CAD build for the part. Positions are in the model's coordinates, mm. Face numbers are marked on the shaded views. A direction names the side the tool comes from. Round coordinates to 2 decimals unless told otherwise and drop trailing zeros. Write each loop counter-clockwise with the first axis right and the second up, starting at its lowest first coordinate (ties: lowest second). Pieces come first, ordered by that corner, then holes. Notation, with made-up numbers: (83.5, 20) - (121.5, 20) arc R28 ccw to (121.5, 46) - close; hole circle Ø2 at (-11.5, 18). An arc over 180 degrees is marked (long way). Answer in a Markdown table with one row per item.
Autodesk Inventor part; units mm, degrees
ref_plane "YZ Plane" through (0, 0, 0) normal (1, 0, 0) x (0, 1, 0)
ref_plane "XZ Plane" through (0, 0, 0) normal (0, 1, 0) x (-1, 0, 0)
ref_plane "XY Plane" through (0, 0, 0) normal (0, 0, 1) x (1, 0, 0)
sketch "Szkic3" plane through (0, 0, 0) normal (0, 1, 0) x (-1, 0, 0)
  line L0 (3.9, 2.7912) -> (3.9, -2.7912)
  line L1 (6.5152, 5.4063) -> (3.9, 2.7912)
  line L2 (8.1306, 5.4063) -> (6.5152, 5.4063)
  line L3 (8.1306, 5.4063) -> (8.1306, 3.0781)
  line L4 (8.1306, -3.0781) -> (8.1306, -5.4064)
  line L5 (8.1306, -5.4064) -> (6.5152, -5.4064)
  line L6 (6.5152, -5.4064) -> (3.9, -2.7912)
  line L7 (8.1306, 3.0781) -> (8.5306, 3.0781)
  line L8 (8.1306, -3.0781) -> (8.5306, -3.0781)
  line L9 (8.5306, -3.0781) -> (12.0661, -6.6136)
  line L10 (8.5306, 3.0781) -> (12.0661, 6.6136)
  line L11 (12.0661, -6.6136) -> (12.0661, -12.6136)
  line L12 (12.0661, 6.6136) -> (12.0661, 12.6136)
  line L13 (12.0661, 12.6136) -> (16.0661, 12.6136)
  line L14 (12.0661, -12.6136) -> (16.0661, -12.6136)
  line L15 (16.0661, -12.6136) -> (16.0661, 12.6136)
  point P0 (8.1306, 4.2422)
  dimension "d85" = 5.5823
  dimension "d88" = 135
  dimension "d89" = 135
  dimension "d90" = 1.6154
  dimension "d91" = 2.6152
  dimension "d92" = 2.3282
  dimension "d99" = 0.4
  dimension "d100" = 5
  dimension "d101" = 135
  dimension "d102" = 5
  dimension "d103" = 135
  dimension "d114" = 180
  dimension "d115" = 6
  dimension "d116" = 6
  dimension "d117" = 4
  dimension "d118" = 4
extrude "Wyciągnięcie proste1" add sketch "Szkic3" along normal blind 24
sketch "Szkic13" plane through (-16.0661, 0, -12.6136) normal (-1, 0, 0) x (0, 0, 1)
  line L0 (12.6136, 15.06) -> (15.2636, 13.53)
  line L1 (15.2636, 13.53) -> (15.2636, 10.47)
  line L2 (15.2636, 10.47) -> (12.6136, 8.94)
  line L3 (12.6136, 8.94) -> (9.9636, 10.47)
  line L4 (9.9636, 10.47) -> (9.9636, 13.53)
  line L5 (9.9636, 13.53) -> (12.6136, 15.06)
  line L6 (0, 24) -> (25.2273, 24)
  line L7 (25.2273, 0) -> (25.2273, 24)
  point P0 (12.6136, 0)
  point P1 (12.6136, 12)
  point P2 (12.6136, 24)
  dimension "d119" = 12
  dimension "d120" = 12.6136
  dimension "d121" = 5.3
extrude "Wyciągnięcie proste5" cut sketch "Szkic13" against normal blind 6
sketch "Szkic14" plane through (-10.0661, 0, -12.6136) normal (-1, 0, 0) x (0, 0, 1)
  circle A0 centre (12.6136, 12) radius 1.7
  point P0 (12.6136, 0)
  dimension "d124" = 3.4
extrude "Wyciągnięcie proste6" cut sketch "Szkic14" against normal through all
sketch "Szkic15" plane through (0, 0, 0) normal (0, 0, 1) x (1, 0, 0)
  line L0 (-3.9, 13.7) -> (-3.9, 10.3)
  line L1 (-10.0661, 10.3) -> (-10.0661, 13.7)
  point P0 (0, 0)
  dimension "d127" = 6.1661
sketch "Szkic16" plane through (-16.0661, 0, -12.6136) normal (-1, 0, 0) x (0, 0, 1)
  point P0 (12.6136, 0)
sketch "Szkic17" plane through (-16.0661, 0, -12.6136) normal (-1, 0, 0) x (0, 0, 1)
  line L0 (25.2273, 0) -> (25.2273, 24)
  line L1 (0, 24) -> (25.2273, 24)
  line L2 (25.2273, 0) -> (18.7273, 0)
  line L3 (18.7273, 0) -> (18.7273, 24)
  line L4 (18.7273, 24) -> (25.2273, 24)
  line L5 (25.2273, 24) -> (25.2273, 0)
  line L6 (9.5355, 24) -> (6, 24)
  line L7 (6.5, 24) -> (0, 24)
  line L8 (0, 24) -> (0, 0)
  line L9 (0, 0) -> (6.5, 0)
  line L10 (6.5, 0) -> (6.5, 24)
  line L11 (0, 0) -> (0, 24)
  line L12 (0, 0) -> (25.2273, 0)
  point P0 (12.6136, 0)
  dimension "d128" = 6.5
  dimension "d129" = 6.5
extrude "Wyciągnięcie proste7" add sketch "Szkic17" along normal blind 10 contours L2 L3 L1 L0 | L9 L8 L1 L10
sketch "Szkic18" plane through (-26.0661, 0, -12.6136) normal (-1, 0, 0) x (0, 0, 1)
  circle A0 centre (23.0973, 2) radius 0.85
  line L0 (25.2273, 0) -> (25.2273, 24)
  line L1 (18.7273, 0) -> (25.2273, 0)
  circle A1 centre (2.13, 2) radius 0.85
  line L2 (0, 0) -> (6.5, 0)
  line L3 (0, 24) -> (0, 0)
  circle A2 centre (23.0973, 14.5) radius 0.85
  circle A3 centre (2.13, 14.5) radius 0.85
  line L4 (2.13, 4.5) -> (0, 4.5)
  line L5 (0, 4.5) -> (0, 12)
  line L6 (0, 12) -> (2.13, 12)
  line L7 (2.13, 12) -> (2.13, 4.5)
  line L8 (25.2273, 0) -> (25.2273, 24)
  line L9 (25.2273, 4.5) -> (23.0973, 4.5)
  line L10 (23.0973, 4.5) -> (23.0973, 12)
  line L11 (23.0973, 12) -> (25.2273, 12)
  line L12 (25.2273, 12) -> (25.2273, 4.5)
  point P0 (12.6136, 0)
  point P1 (21.9773, 0)
  point P2 (0, 8.25)
  point P3 (2.13, 8.25)
  point P4 (0, 12)
  point P5 (0, 4.5)
  dimension "d132" = 1.7
  dimension "d133" = 2.13
  dimension "d134" = 2
  dimension "d135" = 2
  dimension "d136" = 2.13
  dimension "d137" = 1.7
  dimension "d138" = 1.7
  dimension "d139" = 12.5
  dimension "d140" = 2.13
  dimension "d141" = 1.7
  dimension "d142" = 2.13
  dimension "d143" = 12.5
  dimension "d144" = 2.5
  dimension "d145" = 2.5
  dimension "d147" = 2.13
  dimension "d148" = 2.5
  dimension "d149" = 2.5
  dimension "d150" = 2.13
extrude "Wyciągnięcie proste8" add sketch "Szkic18" along normal blind 3 contours L9 L10 L11 L0 | L6 L7 L4 L3
extrude "Wyciągnięcie proste9" cut sketch "Szkic18" against normal blind 5 contours A0 | A1 | A2 | A3
fillet "Zaokrąglenie1" radius 2 14 edges at (-16.0661, 12, 6.1136) (-16.0661, 12, -6.1136) (-26.0661, 12, -6.1136) (-26.0661, 12, 6.1136) (-12.0661, 12, 12.6136) (-12.0661, 12, -12.6136) (-19.0661, 0, -12.6136) (-12.0661, 0, -9.6136) (-19.0661, 24, -12.6136) (-12.0661, 24, -9.6136) (-12.0661, 24, 9.6136) (-19.0661, 24, 12.6136) (-12.0661, 0, 9.6136) (-19.0661, 0, 12.6136)
properties part number "Montaż_kamery_Drukowanie 3D"
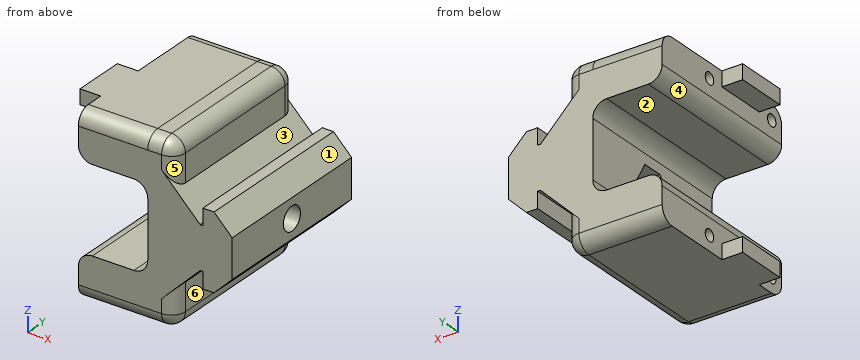
Q1. Pull direction X, two halves, no side cores. Call the marked faces 1, 2 and 3: released by +X, released by -X, zero draft, split by the parting line, or undercut.
Computed:
| item | result |
|---|---|
| face 1 | released by +X |
| face 2 | zero draft |
| face 3 | undercut |
Q2. Saw through at C-C on x = -7. List the corners of the cut face in (y, z).
Computed:
| item | result |
|---|---|
| outline | (0, -5.41) - (24, -5.41) - (24, 5.41) - (0, 5.41) - close; hole circle Ø3.4 at (12, 0) |
Q3. Saw through at D-D on x = -13.25. List the corners of the cut face in (y, z), then the cut area to 3 significant figures.
Computed:
| item | result |
|---|---|
| outline | (0, -7.8) - (0.17, -7.8) - (0.17, -10.61) arc R1.83 ccw to (2, -12.44) - (22, -12.44) arc R1.83 ccw to (23.83, -10.61) - (23.83, -7.8) - (24, -7.8) - (24, 7.8) - (23.83, 7.8) - (23.83, 10.61) arc R1.83 ccw to (22, 12.44) - (2, 12.44) arc R1.83 ccw to (0.17, 10.61) - (0.17, 7.8) - (0, 7.8) - close; hole (8.94, 0) - (10.47, -2.65) - (13.53, -2.65) - (15.06, 0) - (13.53, 2.65) - (10.47, 2.65) - close |
| area | 567 mm2 |
Q4. Saw through at B-B on z = -0.75. List the corners of the cut face in (x, y), then the cut area to 3 significant figures.
Computed:
| item | result |
|---|---|
| outline | (-16.07, 0) - (-3.9, 0) - (-3.9, 10.47) - (-10.07, 10.47) - (-10.07, 9.37) - (-16.07, 9.37) - close; (-16.07, 14.63) - (-10.07, 14.63) - (-10.07, 13.53) - (-3.9, 13.53) - (-3.9, 24) - (-16.07, 24) - close |
| area | 242 mm2 |
Q5. Drill centre lines: line 1 (Y direction, x = -6.75, z = 0); line 2 (Y direction, x = -22.5, z = 9.75); line 3 (Z direction, x = -20.25, y = 13). Where is each one in solid material? Low to high.
Computed:
| item | result |
|---|---|
| line 1 | y = 0 to 10.3, 13.7 to 24 |
| line 2 | y = 0 to 1.57, 2.43 to 14.07, 14.93 to 24 |
| line 3 | z = -12.61 to -6.11, 6.11 to 12.61 |
Q6. 3-axis set-ups, long thin cutter, end or side, ignore diameter. For the marked faces 4, 5 and 6: which of +Z, -Z, +X, -X, +Y, -Y reach the whole face in a straight line?
Computed:
| item | result |
|---|---|
| face 4 | -X, +Y, -Y |
| face 5 | +Z, +X, -Y |
| face 6 | -Z, +X, +Y, -Y |
Q7. Flat gauge pins, fed straight in: pin 1 (1 mm diameter, centred on y = 13, z = 11.5, fed in from +X); pin 2 (3.5 mm diameter, centred on y = 15.5, z = -10.5, fed in from -X); pin 3 (6.5 mm diameter, centred on y = 10.5, z = -2, fed in from -X). Where does each tip first touch, or does it go through?
Computed:
| item | result |
|---|---|
| pin 1 | stops at x = -12.1 |
| pin 2 | stops at x = -26.07 |
| pin 3 | stops at x = -16.42 |
Q8. Saw through at A-A on x = -19.5. List the corners of the cut face in (y, z), then the cut area to 3 significant figures.
Computed:
| item | result |
|---|---|
| outline | (0, -10.61) arc R2 ccw to (2, -12.61) - (22, -12.61) arc R2 ccw to (24, -10.61) - (24, -6.11) - (0, -6.11) - close; (0, 6.11) - (24, 6.11) - (24, 10.61) arc R2 ccw to (22, 12.61) - (2, 12.61) arc R2 ccw to (0, 10.61) - close |
| area | 309 mm2 |
